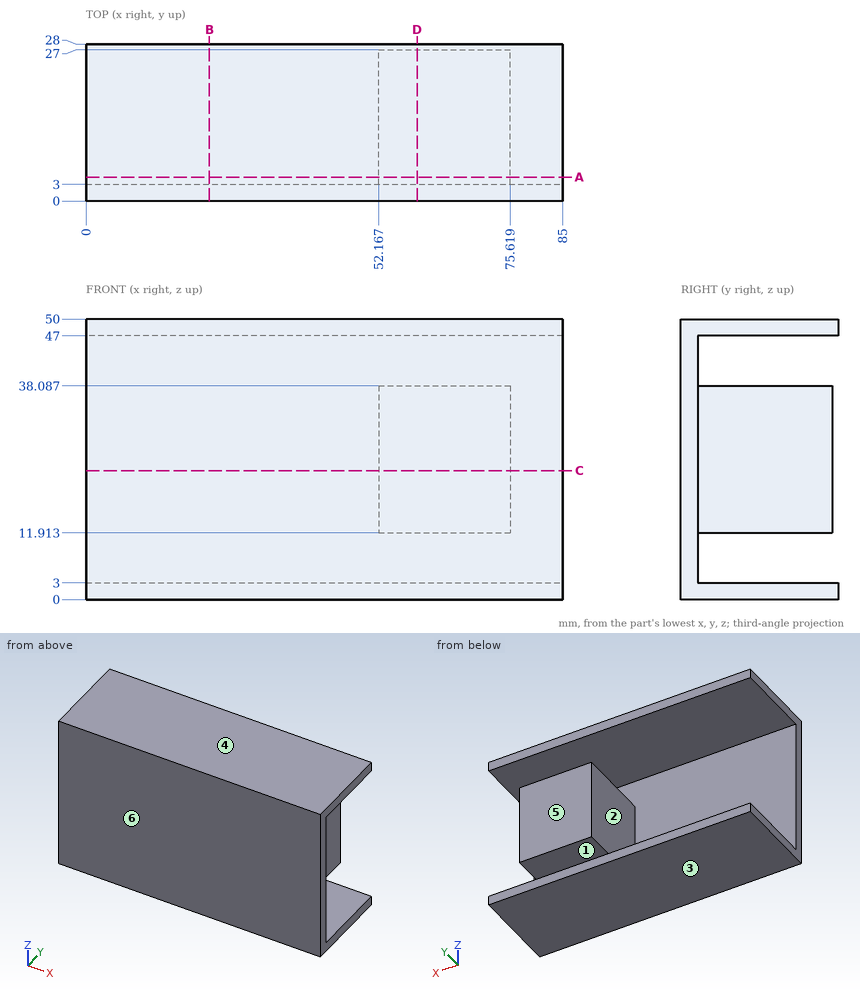
Job drawing, mm, ordinate dimensions from the low corner. One solid piece. A direction names the side the tool comes from. Round coordinates to 2 decimals unless told otherwise and drop trailing zeros. Loops run counter-clockwise (first coordinate to the right, second up) from the corner with the lowest first, then second, coordinate; pieces in that order, holes last.
(1) Drop flat-ended pins along their axis: pin 1 (12 mm diameter, centred on x = 46, z = 26.5, fed in from +Y); pin 2 (13 mm diameter, centred on x = 48, z = 14, fed in from +Y); pin 3 (12 mm diameter, centred on y = 13.5, z = 15.5, fed in from -X). Give the stop position or say it passes through.
(2) Cut at B-B (x = 22). Give the cut face in (y, z), plus the area to 3 significant figures.
(3) Cut at D-D (x = 59). Give the cut face in (y, z).
(4) Wall check: line 1 along Z through (x, y) = (64, 26.5); line 2 along Z through (x, y) = (39.5, 15.25); line 3 along X through (y, z) = (13.75, 31). Give the ranges that are in metal, low to high.
(5) Cut at A-A (y = 4.25). Give the cut face in (x, z).
(6) Two-plate mould, pull along Z, no slides. Class the marked faces 4, 5 and 6: +Z half, -Z half, draft (parallel to the pull), parting line (faces both ways), or undercut.
(7) Cut at C-C (z = 23). Give the cut face in (x, y).
(8) Which spindle directions (+Z, -Z, +X, -X, +Y, -Y) get a long thin tool onto all of the face, cutting with end or side? Do the marked faces 1, 2 and 3. Say none if no direction does.
Findings below:
1. pin 1: stops at y = 3
1. pin 2: stops at y = 27
1. pin 3: stops at x = 52.17
2. outline: (0, 0) - (28, 0) - (28, 3) - (3, 3) - (3, 47) - (28, 47) - (28, 50) - (0, 50) - close
2. area: 300 mm2
3. outline: (0, 0) - (28, 0) - (28, 3) - (3, 3) - (3, 11.91) - (27, 11.91) - (27, 38.09) - (3, 38.09) - (3, 47) - (28, 47) - (28, 50) - (0, 50) - close
4. line 1: z = 0 to 3, 11.91 to 38.09, 47 to 50
4. line 2: z = 0 to 3, 47 to 50
4. line 3: x = 52.17 to 75.62
5. outline: (0, 0) - (85, 0) - (85, 3) - (0, 3) - close; (0, 47) - (85, 47) - (85, 50) - (0, 50) - close; (52.17, 11.91) - (75.62, 11.91) - (75.62, 38.09) - (52.17, 38.09) - close
6. face 4: +Z half
6. face 5: undercut
6. face 6: draft
7. outline: (0, 0) - (85, 0) - (85, 3) - (75.62, 3) - (75.62, 27) - (52.17, 27) - (52.17, 3) - (0, 3) - close
8. face 1: +X, -X, +Y
8. face 2: -X, +Y
8. face 3: -Z, +X, -X, +Y, -Y
